Verification items for the finished model (mm, model axes). Face numbers are marked on the shaded views. A direction names the side the tool comes from. Give positions to 0.01 mm unless a question says otherwise; leave off trailing zeros. Order: outer loops, then holes, each group sorted by start corner. A loop starts at its lowest first (then second) coordinate and runs counter-clockwise, first axis right, second up. Notation, with made-up numbers: (62.5, 52.5) - (84.5, 52.5) arc R19 cw to (84.5, 63.5) - close; hole circle Ø6 at (47, 64). An arc over 180 degrees is marked (long way). Answer as a JSON object with one key per item and string values. Group by question number.
(1) Mould release check, pull along Y, two halves, no side actions. Record for the marked faces 5, 6, 7 and 8: +Y half, -Y half, draft (parallel to the pull), parting line (faces both ways), or undercut.
(2) Section check C-C (z = 15.5). Record the boundary of the cut face in (x, y).
(3) Section check B-B (y = -2.5). Record the boundary of the cut face in (x, z).
(4) Access from +Z, -Z, +X, -X, +Y, -Y to the whole of each face (thin tool, end or side, straight path). Record for the marked faces 1, 2, 3 and 4.
(5) Section check A-A (x = 0). Record the boundary of the cut face in (y, z), then the cut area to 3 significant figures.
(6) Section check D-D (x = 5.5). Record the boundary of the cut face in (y, z).
(7) Thickness scan on line 1 (X direction, y = 2.25, z = 7); line 2 (Y direction, x = -7, z = 25); line 3 (X direction, y = 12.5, z = 19.75). Record the ranges inside material, lowest first.
(8) Depth check by flat-ended pin: pin 1 Ø12 at (x, y) = (-2, -2) entering from +Z; pin 2 Ø5.5 at (x, z) = (-0.5, 21) entering from -Y. Enter the tip coordinate at first touch or a pass-through.
Autodesk Inventor part; units mm, degrees
ref_plane "YZ Plane" through (0, 0, 0) normal (1, 0, 0) x (0, 1, 0)
ref_plane "XZ Plane" through (0, 0, 0) normal (0, 1, 0) x (-1, 0, 0)
ref_plane "XY Plane" through (0, 0, 0) normal (0, 0, 1) x (1, 0, 0)
sketch "스케치1" plane through (0, 0, 0) normal (0, 0, 1) x (1, 0, 0)
  line L0 (12.5, -15) -> (-12.5, -15)
  line L1 (-12.5, -15) -> (-12.5, 15)
  line L2 (-12.5, 15) -> (12.5, 15)
  line L3 (12.5, 15) -> (12.5, -15)
  line L4 (12.5, -15) -> (-12.5, 15) construction
  line L5 (-12.5, -15) -> (12.5, 15) construction
  point P0 (0, 0)
  dimension "d0" = 25
  dimension "d1" = 30
extrude "돌출1" add sketch "스케치1" along normal blind 5
sketch "스케치2" plane through (0, 0, 5) normal (0, 0, 1) x (1, 0, 0)
  line L0 (12.5, 15) -> (-12.5, 15)
  line L1 (12.5, -15) -> (12.5, 15)
  line L2 (-12.5, 15) -> (12.5, 15)
  line L3 (12.5, 15) -> (12.5, 10)
  line L4 (12.5, 10) -> (-12.5, 10)
  line L5 (-12.5, 10) -> (-12.5, 15)
  point P0 (0, 0)
  dimension "d4" = 5
extrude "돌출2" add sketch "스케치2" along normal blind 25
sketch "스케치3" plane through (0, 0, 5) normal (0, 0, 1) x (1, 0, 0)
  line L0 (0, -3) -> (0, 3) construction
  line L1 (3.5, -3) -> (3.5, 3)
  line L2 (-3.5, 3) -> (-3.5, -3)
  arc A0 (-3.5, -3) -> (3.5, -3) centre (0, -3) ccw
  arc A1 (3.5, 3) -> (-3.5, 3) centre (0, 3) ccw
  point P0 (0, 0)
  dimension "d7" = 3
  dimension "d8" = 7
extrude "돌출3" cut sketch "스케치3" against normal through all
sketch "스케치4" plane through (-12.5, 10, 5) normal (0, -1, 0) x (1, 0, 0)
  line L0 (25, 0) -> (0, 0)
  line L1 (0, 0) -> (12.5, 0)
  line L2 (12.5, 7) -> (12.5, 13) construction
  line L3 (16, 7) -> (16, 13)
  line L4 (9, 13) -> (9, 7)
  arc A0 (9, 7) -> (16, 7) centre (12.5, 7) ccw
  arc A1 (16, 13) -> (9, 13) centre (12.5, 13) ccw
  point P0 (12.5, -5)
  dimension "d14" = 7
extrude "돌출4" cut sketch "스케치4" against normal through all
sketch "스케치5" plane through (-12.5, -15, 0) normal (-1, 0, 0) x (0, 0, 1)
  line L0 (0, 30) -> (0, 0)
  line L1 (0, 0) -> (5, 0)
  line L2 (5, 25) -> (5, 0)
  line L3 (5, 25) -> (30, 25)
  line L4 (30, 30) -> (30, 25)
  line L5 (0, 30) -> (30, 30)
  line L6 (0, 0) -> (0, 30)
  line L7 (0, 30) -> (30, 30)
  line L8 (0, 0) -> (30, 0)
  line L9 (30, 0) -> (30, 30)
  line L10 (30, 30) -> (0, 30)
  line L11 (0, 30) -> (0, 0)
  line L12 (5, 0) -> (6, 0)
  line L13 (30, 25) -> (30, 24)
  line L14 (30, 24) -> (6, 0)
  circle A0 centre (30, 0) radius 24
  point P0 (0, 15)
  dimension "d17" = 1
  dimension "d18" = 1
extrude "돌출5" add sketch "스케치5" against normal blind 3 contours L2 L3 L9 A0 L8
sketch "스케치6" plane through (12.5, -15, 0) normal (1, 0, 0) x (0, 0, -1)
  line L0 (-30, 25) -> (-5, 25)
  line L1 (-30, 25) -> (-30, 24)
  arc A0 (-6, 0) -> (-30, 24) centre (-30, 0) ccw
  line L2 (-6, 0) -> (-5, 0)
  line L3 (-5, 25) -> (-5, 0)
  point P0 (0, 15)
extrude "돌출6" add sketch "스케치6" against normal blind 3
fillet "모깎기1" radius 2 8 edges at (-11, -15, 6) (0, -15, 5) (11, -15, 6) (0, 10, 30) (-11, 9, 30) (11, 9, 30) (0, 10, 5) (0, 15, 0)
properties part number "braket2"
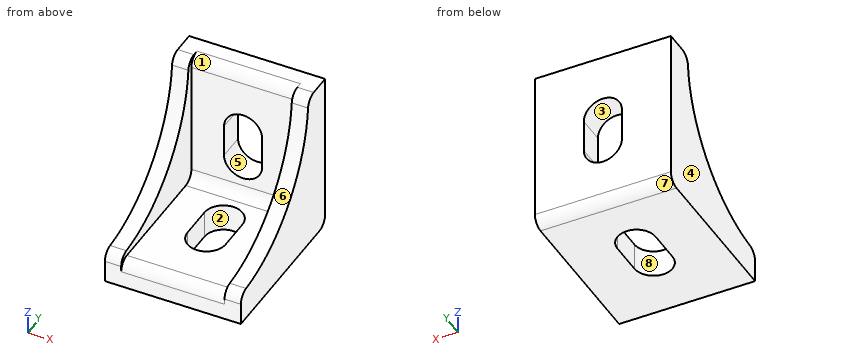
Solutions:
{
 "1": {"face 5": "draft", "face 6": "-Y half", "face 7": "+Y half", "face 8": "undercut"},
 "2": {"outline": "(-12.5, 4.12) - (-9.5, 4.12) - (-9.5, 10) - (-3.5, 10) - (-3.5, 15) - (-12.5, 15) - close; (3.5, 10) - (9.5, 10) - (9.5, 4.12) - (12.5, 4.12) - (12.5, 15) - (3.5, 15) - close"},
 "3": {"outline": "(-12.5, 0) - (-3.5, 0) - (-3.5, 5) - (-9.5, 5) - (-9.5, 9.51) - (-12.5, 9.51) - close; (3.5, 0) - (12.5, 0) - (12.5, 9.51) - (9.5, 9.51) - (9.5, 5) - (3.5, 5) - close"},
 "4": {"face 1": "+Z, -Y", "face 2": "+Z, -Z", "face 3": "+Y, -Y", "face 4": "+Z, -Z, -X, +Y, -Y"},
 "5": {"outline": "(-15, 0) - (-6.5, 0) - (-6.5, 5) - (-13, 5) arc R2 ccw to (-15, 3) - close; (6.5, 0) - (13, 0) arc R2 ccw to (15, 2) - (15, 8.5) - (10, 8.5) - (10, 7) arc R2 cw to (8, 5) - (6.5, 5) - close; (10, 21.5) - (15, 21.5) - (15, 30) - (12, 30) arc R2 ccw to (10, 28) - close", "area": "143 mm2"},
 "6": {"outline": "(-15, 0) - (13, 0) arc R2 ccw to (15, 2) - (15, 30) - (12, 30) arc R2 ccw to (10, 28) - (10, 7) arc R2 cw to (8, 5) - (-13, 5) arc R2 ccw to (-15, 3) - close"},
 "7": {"line 1": "x = -12.5 to -9.5, 9.5 to 12.5", "line 2": "y = 10 to 15", "line 3": "x = -12.5 to -3.03, 3.03 to 12.5"},
 "8": {"pin 1": "stops at z = 5", "pin 2": "stops at y = 10"}
}
